from build123d import *

# Parameters (mm, degrees)
BOSS_EXTRUDE1_DEPTH     = 40
SKETCH3_W               = 20
SKETCH3_H               = 15
CUT_EXTRUDE1_DEPTH      = 10
CUT_EXTRUDE5_DEPTH      = 41
CUT_EXTRUDE5_DEPTH_BACK = 10


with BuildPart() as part:
    # Sketch1 → Boss-Extrude1 (new body)
    with BuildSketch(Plane.XY):
        with BuildLine():
            Line((20, 0), (50, 0))
            Line((50, 0), (50, 10))
            Line((50, 10), (20, 10))
            ThreePointArc((20, 10), (12.928932188, 12.928932188), (10, 20))
            Line((10, 20), (10, 50))
            Line((10, 50), (0, 50))
            Line((0, 50), (0, 20))
            ThreePointArc((0, 20), (5.857864376, 5.857864376), (20, 0))
        make_face()
    extrude(amount=-BOSS_EXTRUDE1_DEPTH)

    # Sketch3 → Cut-Extrude1 (cut)
    with BuildSketch(Plane(origin=(10, 0, 0), x_dir=(0, 0, -1), z_dir=(1, 0, 0))):
        with Locations((10, 42.5)):
            Rectangle(SKETCH3_W, SKETCH3_H)
    extrude(amount=-CUT_EXTRUDE1_DEPTH, mode=Mode.SUBTRACT)

    # Sketch4 → Cut-Extrude5 (cut, two sides)
    with BuildSketch(Plane(origin=(0, 10, 0), x_dir=(1, 0, 0), z_dir=(0, 1, 0))) as cut_extrude5_sk:
        with BuildLine():
            Line((174.127122105, 27.5), (50, 27.5))
            Line((50, 27.5), (35, 27.5))
            Line((35, 27.5), (35, 27.448852076))
            ThreePointArc((35, 27.448852076), (27.551147924, 20), (35, 12.551147924))
            Line((35, 12.551147924), (35, 12.5))
            Line((35, 12.5), (50, 12.5))
            Line((50, 12.5), (174.127122105, 12.5))
            Line((174.127122105, 12.5), (422.381366315, 12.5))
            Line((422.381366315, 12.5), (422.381366315, 27.5))
            Line((422.381366315, 27.5), (174.127122105, 27.5))
        make_face()
    extrude(amount=CUT_EXTRUDE5_DEPTH, mode=Mode.SUBTRACT)
    extrude(cut_extrude5_sk.sketch, amount=-CUT_EXTRUDE5_DEPTH_BACK, mode=Mode.SUBTRACT)


solid = part.part
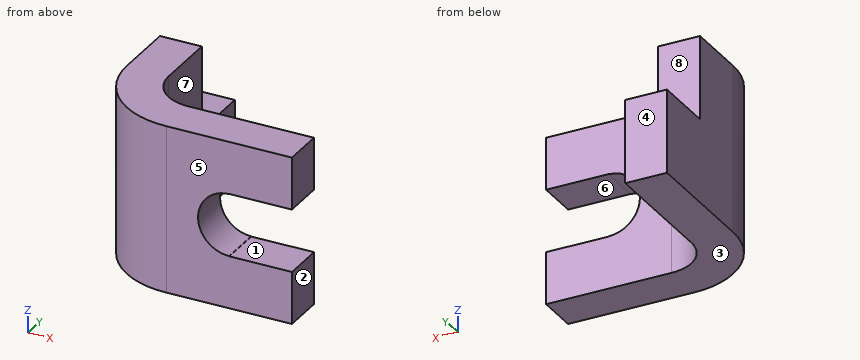
CAD build for the part. Positions are in the model's coordinates, mm. Face numbers are marked on the shaded views. A direction names the side the tool comes from. Round coordinates to 2 decimals unless told otherwise and drop trailing zeros. Write each loop counter-clockwise with the first axis right and the second up, starting at its lowest first coordinate (ties: lowest second). Pieces come first, ordered by that corner, then holes.
(1) Slice it at B-B, the plane z = -6.5. Write the cut outline in (x, y).
(2) Mould opens along Z. For the marked faces 1, 2 and 3 say: pulls with the +Z half, pulls with the -Z half, needs draft (parallel to the pull), parting line crosses it, or undercut.
(3) Drop flat-ended pins along their axis: P1, Ø1.5, axis at y = 27.5, z = -31.5, coming from the +X side; P2, Ø12, axis at x = 33, z = -13, coming from the +Y side; P3, Ø3, axis at x = 5.5, z = -8.5, coming from the +Y side. Give the stop position or say it passes through.
(4) 3-axis set-ups, long thin cutter, end or side, ignore diameter. For the marked faces 4, 5, 6, 7 and 8: which of +Z, -Z, +X, -X, +Y, -Y reach the whole face in a straight line?
(5) Probe line 1 along Y through (x, z) = (31, -28); line 2 along Z through (x, y) = (4.5, 38). List the from-to ranges inside material, lowest first.
(6) Slice it at C-C, the plane y = 24. Write the cut outline in (x, z).
(7) Slice it at A-A, the plane x = 36. Write the cut outline in (y, z), and give its area (3 significant figures).
From the geometry:
1. outline: (0, 20) arc R20 ccw to (20, 0) - (50, 0) - (50, 10) - (20, 10) arc R10 cw to (10, 20) - (10, 35) - (0, 35) - close
2. face 1: undercut
2. face 2: needs draft
2. face 3: pulls with the -Z half
3. P1: stops at x = 10
3. P2: stops at y = 10
3. P3: stops at y = 35
4. face 4: +Z, -Z, +X, -X, +Y
4. face 5: +Z, -Z, +X, -X, -Y
4. face 6: +X, +Y, -Y
4. face 7: +Z, -Z, +X, +Y
4. face 8: +Z, +X, -X, +Y
5. line 1: y = 0 to 10
5. line 2: z = -40 to -20
6. outline: (0, -40) - (10, -40) - (10, 0) - (0, 0) - close
7. outline: (0, -40) - (10, -40) - (10, -27.5) - (0, -27.5) - close; (0, -12.5) - (10, -12.5) - (10, 0) - (0, 0) - close
7. area: 250 mm2
